Source: CAD feature listing. Evaluate the final solid. Frame: model axes, mm. A direction names the side the tool comes from. Round coordinates to 2 decimals unless told otherwise and drop trailing zeros. Loops run counter-clockwise (first coordinate to the right, second up) from the corner with the lowest first, then second, coordinate; pieces in that order, holes last. Notation, with made-up numbers: (34.5, 18) - (52.5, 18) arc R14 cw to (52.5, 28) - close; hole circle Ø10 at (-35, 36.25). An arc over 180 degrees is marked (long way). One line per question, with ' | ' between items. Start each with the question number.
1. Mould query, pull axis Z, two halves, no side actions, for faces 6 (the flat face through (824, 74, -210)), 7 (the flat face through (799, 99, -200)), 8 (the flat face through (48, 904, 0)). Classes: pulls with the +Z half, pulls with the -Z half, needs draft (parallel to the pull), parting line crosses it, or undercut.
2. Pin query (flat end, axial travel): pin 1 (2.5 mm diameter, centred on x = 52.5, y = 461.5, fed in from -Z). Return the tip coordinate at first contact, or that it passes through.
3. Cut plane C-C (y = 360). Return loops of the section in (x, z), then the cut area to 4 significant figures.
4. Cut plane B-B (z = -58.5). Return loops of the section in (x, y), then the cut area to 3 significant figures.
5. Cut plane A-A (x = 123). Return loops of the section in (y, z).
6. Cut plane D-D (z = -164). Return loops of the section in (x, y).
7. Ray query, line 1 (Y direction, x = 443.5, z = -78); line 2 (Y direction, x = 506.5, z = -110); line 3 (Y direction, x = 392.5, z = -198). Return the intervals inside material, ascending.
8. Access query for faces 1 (the flat face through (799, 1699, -200)), 2 (the flat face through (25, 910, -200)), 3 (the flat face through (444, 1800, -104)), 4 (the flat face through (444, 900, -130)), 5 (the flat face through (900, 887, -104)). Directions: +Z, -Z, +X, -X, +Y, -Y. A direction counts if a zero-diameter tool reaches every point of the face in a straight line with its end or side. Return the directions, or none.
```python
from build123d import *

# Parameters (mm, degrees)
F0_W      = 900
F0_H      = 1800
F0_W_2    = 800
F0_H_2    = 50
F1_DEPTH  = 200
F2_W      = 800
F2_H      = 30
F3_DEPTH  = 50
F4_W      = 800
F4_H      = 70
F5_DEPTH  = 50
F6_W      = 150
F6_H      = 150
F7_DEPTH  = 10
F9_DEPTH  = 825
F11_DEPTH = 825


with BuildPart() as f1:
    # F0 (on Top) → F1 (new body)
    with BuildSketch(Plane.XY):
        with Locations((450, 900)):
            Rectangle(F0_W, F0_H)
        Polygon((850, 50), (50, 50), (50, 875), (50, 925), (50, 1750), (850, 1750), (850, 925), (850, 875), align=None, mode=Mode.SUBTRACT)
        with Locations((450, 900)):
            Rectangle(F0_W_2, F0_H_2)
    extrude(amount=-F1_DEPTH)

    # F2 (on face) → F3 (cut, through all)
    with BuildSketch(Plane.XZ.offset(-875)):
        with Locations((450, -15)):
            Rectangle(F2_W, F2_H)
    extrude(amount=-F3_DEPTH, mode=Mode.SUBTRACT)

    # F4 (on face) → F5 (cut, through all)
    with BuildSketch(Plane.XZ.offset(-875)):
        with Locations((450, -165)):
            Rectangle(F4_W, F4_H)
    extrude(amount=-F5_DEPTH, mode=Mode.SUBTRACT)

    # F6 (on face) → F7 (join)
    with BuildSketch(Plane(origin=(0, 0, -200), x_dir=(1, 0, 0), z_dir=(0, 0, -1))):
        with Locations((75, -75)):
            Rectangle(F6_W, F6_H)
        with Locations((825, -75)):
            Rectangle(F6_W, F6_H)
        with Locations((75, -1725)):
            Rectangle(F6_W, F6_H)
        with Locations((825, -1725)):
            Rectangle(F6_W, F6_H)
    extrude(amount=F7_DEPTH)

    # F8 (on face) → F9 (join, through all)
    with BuildSketch(Plane.XZ.offset(-1750)):
        Polygon((100, -30), (50, -30), (50, -80), (55, -80), (55, -35), (100, -35), align=None)
        Polygon((845, -35), (845, -80), (850, -80), (850, -30), (800, -30), (800, -35), align=None)
    extrude(amount=F9_DEPTH)

    # F10 (on face) → F11 (join, through all)
    with BuildSketch(Plane(origin=(0, 50, 0), x_dir=(-1, 0, 0), z_dir=(0, 1, 0))):
        Polygon((-800, -30), (-850, -30), (-850, -80), (-845, -80), (-845, -35), (-800, -35), align=None)
        Polygon((-55, -35), (-55, -80), (-50, -80), (-50, -30), (-100, -30), (-100, -35), align=None)
    extrude(amount=F11_DEPTH)

    # F12 (on face) → F13 (join, up to the next surface of F1)
    with BuildSketch(Plane.YZ.offset(100)):
        Polygon((100, -30), (50, -30), (50, -80), (55, -80), (55, -35), (100, -35), align=None)
    extrude(until=Until.NEXT)

    # F14 (on face) → F15 (join, up to the next surface of F1)
    with BuildSketch(Plane.YZ.offset(100)):
        Polygon((1750, -80), (1750, -30), (1700, -30), (1700, -35), (1745, -35), (1745, -80), align=None)
    extrude(until=Until.NEXT)


solid = f1.part
```
Answers follow:
1) face 6: pulls with the -Z half | face 7: undercut | face 8: pulls with the +Z half
2) pin 1: stops at z = -80
3) outline: (0, -200) - (50, -200) - (50, -80) - (55, -80) - (55, -35) - (100, -35) - (100, -30) - (50, -30) - (50, 0) - (0, 0) - close; (800, -35) - (845, -35) - (845, -80) - (850, -80) - (850, -200) - (900, -200) - (900, 0) - (850, 0) - (850, -30) - (800, -30) - close | area: 20,950 mm2
4) outline: (0, 0) - (900, 0) - (900, 1800) - (0, 1800) - close; hole (55, 50) - (100, 50) - (100, 55) - (845, 55) - (845, 875) - (55, 875) - close; hole (55, 925) - (845, 925) - (845, 1745) - (100, 1745) - (100, 1750) - (55, 1750) - close | area: 324,000 mm2
5) outline: (0, -210) - (150, -210) - (150, -200) - (50, -200) - (50, -80) - (55, -80) - (55, -35) - (100, -35) - (100, -30) - (50, -30) - (50, 0) - (0, 0) - close; (875, -130) - (925, -130) - (925, -30) - (875, -30) - close; (1650, -210) - (1800, -210) - (1800, 0) - (1750, 0) - (1750, -30) - (1700, -30) - (1700, -35) - (1745, -35) - (1745, -80) - (1750, -80) - (1750, -200) - (1650, -200) - close
6) outline: (0, 0) - (900, 0) - (900, 1800) - (0, 1800) - close; hole (50, 50) - (850, 50) - (850, 1750) - (50, 1750) - close
7) line 1: y = 0 to 55, 875 to 925, 1745 to 1800 | line 2: y = 0 to 50, 875 to 925, 1750 to 1800 | line 3: y = 0 to 50, 1750 to 1800
8) face 1: none | face 2: -Z, +X, -X | face 3: +Z, -Z, +X, -X, +Y | face 4: -Z | face 5: +Z, -Z, +X, +Y, -Y
